```python
from build123d import *

# Parameters (mm, degrees)
SKETCH_1_R      = 5
EXTRUDE_1_DEPTH = 10
SCALE_1_SCALE   = 0.2


with BuildPart() as part:
    # 草圖1 → 填料-伸長1 (new body)
    with BuildSketch(Plane(origin=(0, 0, 0), x_dir=(1, 0, 0), z_dir=(0, 1, 0))):
        with BuildLine():
            ThreePointArc((0, -10), (10, 0), (0, 10))
            Line((0, 10), (-10, 10))
            Line((-10, 10), (-10, 5))
            Line((-10, 5), (-15, 5))
            Line((-15, 5), (-15, 10))
            Line((-15, 10), (-25, 10))
            Line((-25, 10), (-25, -10))
            Line((-25, -10), (-15, -10))
            Line((-15, -10), (-15, -5))
            Line((-15, -5), (-10, -5))
            Line((-10, -5), (-10, -10))
            Line((-10, -10), (0, -10))
        make_face()
        Circle(SKETCH_1_R, mode=Mode.SUBTRACT)
    extrude(amount=EXTRUDE_1_DEPTH)


with BuildPart() as part_1:
    # 縮放比例1: scaled about (-9.381191691, 5, 0)
    add(part.part.scale(SCALE_1_SCALE).moved(Location((-7.504953353, 4, 0))))


solid = part_1.part
```
Geometry: final body of the model. Coordinates: model frame, mm. A direction names the side the tool comes from. Coordinates: 2 decimals unless noted, no trailing zeros. Order: outer loops, then holes, each group sorted by start corner. A loop starts at its lowest first (then second) coordinate and runs counter-clockwise, first axis right, second up. Notation, with made-up numbers: (13, 10) -> (36, 10) arc R22 cw to (36, 47) -> close; hole circle Ø2 at (50, 10.5). An arc over 180 degrees is marked (long way). Write each question's results on one line, items separated by ' | '. Start each with the question number.
1) Set-up query: faces 5 (the flat face through (-10, 4, 0)), 6 (the flat face through (-10.505, 5, 1.5)), 7 (the flat face through (-9.505, 5, -1.5)). Return all of +Z, -Z, +X, -X, +Y, -Y with unobstructed straight access to the full face (end or side cutting, diameter ignored); none if empty.
2) Cut plane A-A, the plane z = 0. Output: boundary loops of the cut face in (x, y).
3) Material intervals for line 1 along X through (y, z) = (4.55, 0); line 2 along Z through (x, y) = (-7.5, 5.6); line 3 along Z through (x, y) = (-10, 4.8), sorted ascending.
4) Cut plane B-B, the plane y = 4.2. Output: boundary loops of the cut face in (x, z), and give its area (3 significant figures).
5) Mould query, pull axis X, two halves, no side actions, for faces 1 (the flat face through (-12.505, 5, 0)), 2 (the flat face through (-11, 5, -2)), 3 (the flat face through (-10.505, 5, -1.5)), 4 (the cylindrical face through (-5.505, 4.986, 0.044)). Classes: released by +X, released by -X, zero draft, split by the parting line, or undercut.
6) First-contact query: pin 1 (0.8 mm diameter, centred on y = 5, z = -1.5, fed in from +X); pin 2 (0.5 mm diameter, centred on y = 5, z = 1.5, fed in from +X). Flat tips, straight axial feed; report the tip coordinate or a pass-through.
7) Cut plane C-C, the plane z = -0.6. Output: boundary loops of the cut face in (x, y), and give its area (3 significant figures).
Checks:
1) face 5: +Z, -Z, +X, -X, -Y | face 6: +Z, +Y, -Y | face 7: -Z, +Y, -Y
2) outline: (-12.5, 4) -> (-8.5, 4) -> (-8.5, 6) -> (-12.5, 6) -> close; (-6.5, 4) -> (-5.5, 4) -> (-5.5, 6) -> (-6.5, 6) -> close
3) line 1: -12.5 to -8.5, -6.5 to -5.5 | line 2: -2 to -1, 1 to 2 | line 3: -1 to 1
4) outline: (-12.5, -2) -> (-10.5, -2) -> (-10.5, -1) -> (-9.5, -1) -> (-9.5, -2) -> (-7.5, -2) arc R2 ccw to (-7.5, 2) -> (-9.5, 2) -> (-9.5, 1) -> (-10.5, 1) -> (-10.5, 2) -> (-12.5, 2) -> close; hole circle Ø2 at (-7.5, 0) | area: 21.1 mm^2
5) face 1: released by -X | face 2: zero draft | face 3: undercut | face 4: released by +X
6) pin 1: x = -5.83 | pin 2: x = -5.94
7) outline: (-12.5, 4) -> (-8.3, 4) -> (-8.3, 6) -> (-12.5, 6) -> close; (-6.7, 4) -> (-5.6, 4) -> (-5.6, 6) -> (-6.7, 6) -> close | area: 10.6 mm^2
